Work out the finished part from the listing and answer in its coordinate system (mm). Round coordinates to 2 decimals unless told otherwise and drop trailing zeros. Order: outer loops, then holes, each group sorted by start corner. A loop starts at its lowest first (then second) coordinate and runs counter-clockwise, first axis right, second up. Notation, with made-up numbers: M -34.75,56 L 5.25,56 A31 ccw 5.25,83 Z; hole C 56.25,80.25 d10. An arc over 180 degrees is marked long. Return JSON: item names as keys, results as strings.
from build123d import *

# Parameters (mm, degrees)
SKETCH1_R           = 2.5
SKETCH1_R_2         = 2
SKETCH1_W           = 20
SKETCH1_H           = 6
SKETCH1_W_2         = 10
SKETCH1_W_3         = 6
SKETCH1_H_2         = 15.5
BOSS_EXTRUDE1_DEPTH = 6


with BuildPart() as part:
    # Sketch1 → Boss-Extrude1 (new body)
    with BuildSketch(Plane(origin=(0, 0, 0), x_dir=(1, 0, 0), z_dir=(0, 1, 0))):
        with BuildLine():
            Line((-45, 125.078427477), (-45, 120.078427477))
            Line((-45, 120.078427477), (45, 120.078427477))
            Line((45, 120.078427477), (45, 125.078427477))
            ThreePointArc((45, 125.078427477), (73.284271247, 113.362698724), (85, 85.078427477))
            Line((85, 85.078427477), (75, 85.078427477))
            Line((75, 85.078427477), (75, -89.921572523))
            Line((75, -89.921572523), (85, -89.921572523))
            Line((85, -89.921572523), (85, -116.261318485))
            Line((85, -116.261318485), (70.010138709, -124.471382126))
            Line((70.010138709, -124.471382126), (55.010138709, -124.450192088))
            Line((55.010138709, -124.450192088), (51.474604803, -120.914658182))
            Line((51.474604803, -120.914658182), (28.549864753, -120.914658182))
            Line((28.549864753, -120.914658182), (25.014330847, -124.450192088))
            Line((25.014330847, -124.450192088), (-24.985669153, -124.450192088))
            Line((-24.985669153, -124.450192088), (-28.521203059, -120.914658182))
            Line((-28.521203059, -120.914658182), (-51.44594311, -120.914658182))
            Line((-51.44594311, -120.914658182), (-54.981477016, -124.450192088))
            Line((-54.981477016, -124.450192088), (-69.981477016, -124.450192088))
            Line((-69.981477016, -124.450192088), (-85, -116.261318485))
            Line((-85, -116.261318485), (-85, -89.921572523))
            Line((-85, -89.921572523), (-75, -89.921572523))
            Line((-75, -89.921572523), (-75, 85.078427477))
            Line((-75, 85.078427477), (-85, 85.078427477))
            ThreePointArc((-85, 85.078427477), (-73.284271247, 113.362698724), (-45, 125.078427477))
        make_face()
        with Locations(Location((-45, 85.078427477, 0), (0, 0, 270))):
            Circle(SKETCH1_R, mode=Mode.SUBTRACT)
        with Locations(Location((45, 85.078427477, 0), (0, 0, 270))):
            Circle(SKETCH1_R, mode=Mode.SUBTRACT)
        with Locations(Location((-65.857864376, -110.779436899, 0), (0, 0, 270))):
            Circle(SKETCH1_R, mode=Mode.SUBTRACT)
        with Locations(Location((65.857864376, -110.779436899, 0), (0, 0, 90))):
            Circle(SKETCH1_R, mode=Mode.SUBTRACT)
        with Locations(Location((19.5, 65.078427477, 0), (0, 0, 270))):
            Circle(SKETCH1_R_2, mode=Mode.SUBTRACT)
        with Locations(Location((-19.5, 65.078427477, 0), (0, 0, 270))):
            Circle(SKETCH1_R_2, mode=Mode.SUBTRACT)
        Polygon((50.571600169, 109.810660524), (54.814240856, 114.053301211), (68.95637648, 99.911165587), (64.713735792, 95.6685249), align=None, mode=Mode.SUBTRACT)
        with Locations((0, 113.078427477)):
            Rectangle(SKETCH1_W, SKETCH1_H, mode=Mode.SUBTRACT)
        Polygon((-50.11039508, 110.271865613), (-64.252530704, 96.129729989), (-68.495171391, 100.372370676), (-54.353035767, 114.5145063), align=None, mode=Mode.SUBTRACT)
        with Locations((-39.983573085, -110.414658182)):
            Rectangle(SKETCH1_W_2, SKETCH1_H, mode=Mode.SUBTRACT)
        with Locations((40.012234778, -110.414658182)):
            Rectangle(SKETCH1_W_2, SKETCH1_H, mode=Mode.SUBTRACT)
        with Locations((54, -74.171572523)):
            Rectangle(SKETCH1_W_3, SKETCH1_H_2, mode=Mode.SUBTRACT)
        with Locations((-53.888870578, -74.171572523)):
            Rectangle(SKETCH1_W_3, SKETCH1_H_2, mode=Mode.SUBTRACT)
    extrude(amount=BOSS_EXTRUDE1_DEPTH)


solid = part.part
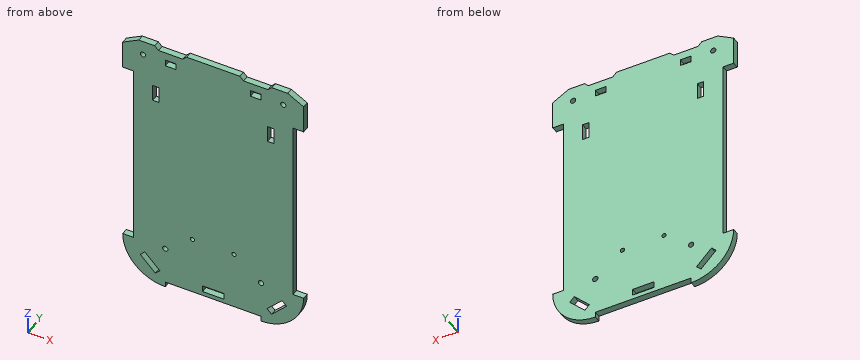
Item 1: Consider line 1 along Z through (x, y) = (52, 5.65); line 2 along Z through (x, y) = (53.5, 2); line 3 along X through (y, z) = (5.35, -11). Determine where each line is inside the solid, lowest interval first. Write a range as [from, to].
Output:
{"line 1": "z = [-124.46, -111.24], [-108.38, 66.42], [81.92, 121.44]", "line 2": "z = [-124.16, -112.74], [-106.88, 66.42], [81.92, 122.94]", "line 3": "x = [-75, 75]"}
Item 2: Find section A-A (z = 73). Determine the outline of the cut face in (x, y), plus the area to 3 significant figures.
Output:
{"outline": "M -75,0 L -56.89,0 L -56.89,6 L -75,6 Z; M -50.89,0 L 51,0 L 51,6 L -50.89,6 Z; M 57,0 L 75,0 L 75,6 L 57,6 Z", "area": "828 mm^2"}
Item 3: Find section B-B (x = 38). Determine the outline of the cut face in (y, z).
Output:
{"outline": "M 0,-120.08 L 6,-120.08 L 6,107.41 L 0,107.41 Z; M 0,113.41 L 6,113.41 L 6,120.91 L 0,120.91 Z"}
Item 4: Find section C-C (x = -13.5). Determine the outline of the cut face in (y, z), plus the area to 3 significant figures.
Output:
{"outline": "M 0,-120.08 L 6,-120.08 L 6,124.45 L 0,124.45 Z", "area": "1,470 mm^2"}
Item 5: Find section D-D (z = 45.5). Determine the outline of the cut face in (x, y).
Output:
{"outline": "M -75,0 L 75,0 L 75,6 L -75,6 Z"}
Item 6: Each of these flat-tipped pins is pushed along its axis until it touches: pin 1 (3 mm diameter, centred on x = 2.5, y = 3, fed in from +Z); pin 2 (3 mm diameter, centred on x = -38, y = 3.5, fed in from -Z); pin 3 (1 mm diameter, centred on y = 3.5, z = 13.5, fed in from +X); pin 4 (4.5 mm diameter, centred on x = -65.86, z = 110.78, fed in from -Y). Where does it stop, or does it pass through?
Output:
{"pin 1": "stops at z = 124.45", "pin 2": "stops at z = -120.08", "pin 3": "stops at x = 75", "pin 4": "passes through"}
